Source: CAD feature listing. Evaluate the final solid. Frame: model axes, mm. Face numbers are marked on the shaded views. Give positions to 0.01 mm unless a question says otherwise; leave off trailing zeros. Write each loop counter-clockwise with the first axis right and the second up, starting at its lowest first coordinate (ties: lowest second). Pieces come first, ordered by that corner, then holes. Notation, with made-up numbers: M 10,59.25 L 30,59.25 A21 ccw 30,96.25 Z; hole C 3.5,64.25 d5. An arc over 180 degrees is marked long. Use CSV: the item, a comma, the result in double quotes. Start each with the question number.
from build123d import *

# Parameters (mm, degrees)
F0_R     = 19.05
F0_R_2   = 13.335
F1_DEPTH = 6.35
F3_D     = 6.35
F4_D     = 6.35


with BuildPart() as f1:
    # F0 (on Front) → F1 (new body, symmetric)
    with BuildSketch(Plane.XZ):
        Circle(F0_R)
        Circle(F0_R_2, mode=Mode.SUBTRACT)
    extrude(amount=F1_DEPTH, both=True)

    # F3 (through all)
    with Locations(Plane(origin=(0, 0, 0), x_dir=(0, 1, 0), z_dir=(-1, 0, 0))):
        with Locations((0, 0)):
            Hole(F3_D / 2)

    # F4 (through all)
    with Locations(Plane.YZ):
        with Locations((0, 0)):
            Hole(F4_D / 2)


solid = f1.part
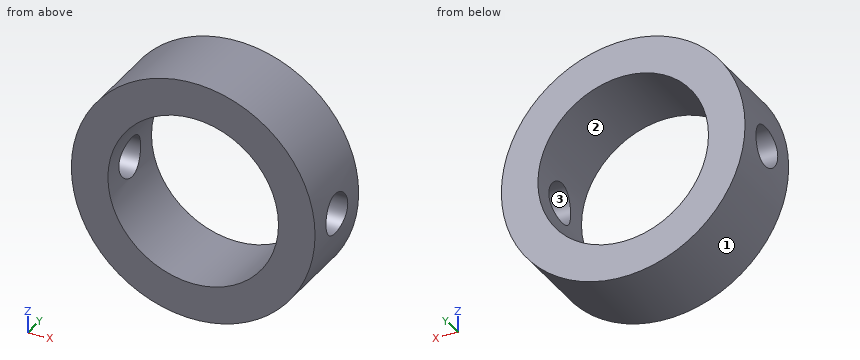
Item 1: Section A-A (z = 0). Return the cut outline in (x, y) (3 decimals).
Item 2: Pull-direction query (X, two-part tool) for the marked faces 1, 2 and 3; classes: released by +X, released by -X, zero draft, split by the parting line, or undercut.
Item 3: Material intervals for probe 1 along Z at (x, y) = (0, -1.5) (3 decimals); probe 2 along Z at (x, y) = (14.75, 0) (3 decimals); probe 3 along X at (y, z) = (4, -9.5), sorted ascending.
Item 4: Section C-C (y = 2). Return the cut outline in (x, z) (3 decimals).
Item 5: Contact query for flat-ended pins moving along their axis: pin 1 Ø16 at (x, z) = (0, 0) entering from +Y; pin 2 Ø3 at (x, y) = (12.5, -0.5) entering from -Z; pin 3 Ø4 at (x, y) = (-10, -1) entering from -Z; pin 4 Ø3 at (x, y) = (11, 0) entering from +Z. Output: stop coordinate, or through.
Item 6: Section B-B (x = 0). Return the cut outline in (y, z) (3 decimals), plus the area to 3 significant figures.
Item 7: Section D-D (y = 5). Return the cut outline in (x, z) (3 decimals), plus the area to 3 significant figures.
Output values:
1,outline,"M -19.05,-6.35 L -13.335,-6.35 L -13.335,-3.175 L -19.05,-3.175 Z; M -19.05,3.175 L -13.335,3.175 L -13.335,6.35 L -19.05,6.35 Z; M 13.335,-6.35 L 19.05,-6.35 L 19.05,-3.175 L 13.335,-3.175 Z; M 13.335,3.175 L 19.05,3.175 L 19.05,6.35 L 13.335,6.35 Z"
2,face 1,"split by the parting line"
2,face 2,"undercut"
2,face 3,"zero draft"
3,probe 1,"z = -19.05 to -13.335, 13.335 to 19.05"
3,probe 2,"z = -12.056 to -3.175, 3.175 to 12.056"
3,probe 3,"x = -16.51 to -9.36, 9.36 to 16.51"
4,outline,"M -18.89,-2.466 A19.05 ccw 18.89,-2.466 L 13.105,-2.466 A13.335 cw -13.105,-2.466 Z; M -18.89,2.466 L -13.105,2.466 A13.335 cw 13.105,2.466 L 18.89,2.466 A19.05 ccw Z"
5,pin 1,"passes through"
5,pin 2,"stops at z = -15.55"
5,pin 3,"stops at z = -17.29"
5,pin 4,"stops at z = 16.51"
6,outline,"M -6.35,-19.05 L 6.35,-19.05 L 6.35,-13.335 L -6.35,-13.335 Z; M -6.35,13.335 L 6.35,13.335 L 6.35,19.05 L -6.35,19.05 Z"
6,area,"145 mm2"
7,outline,"C 0,0 d38.1; hole C 0,0 d26.67"
7,area,"581 mm2"
